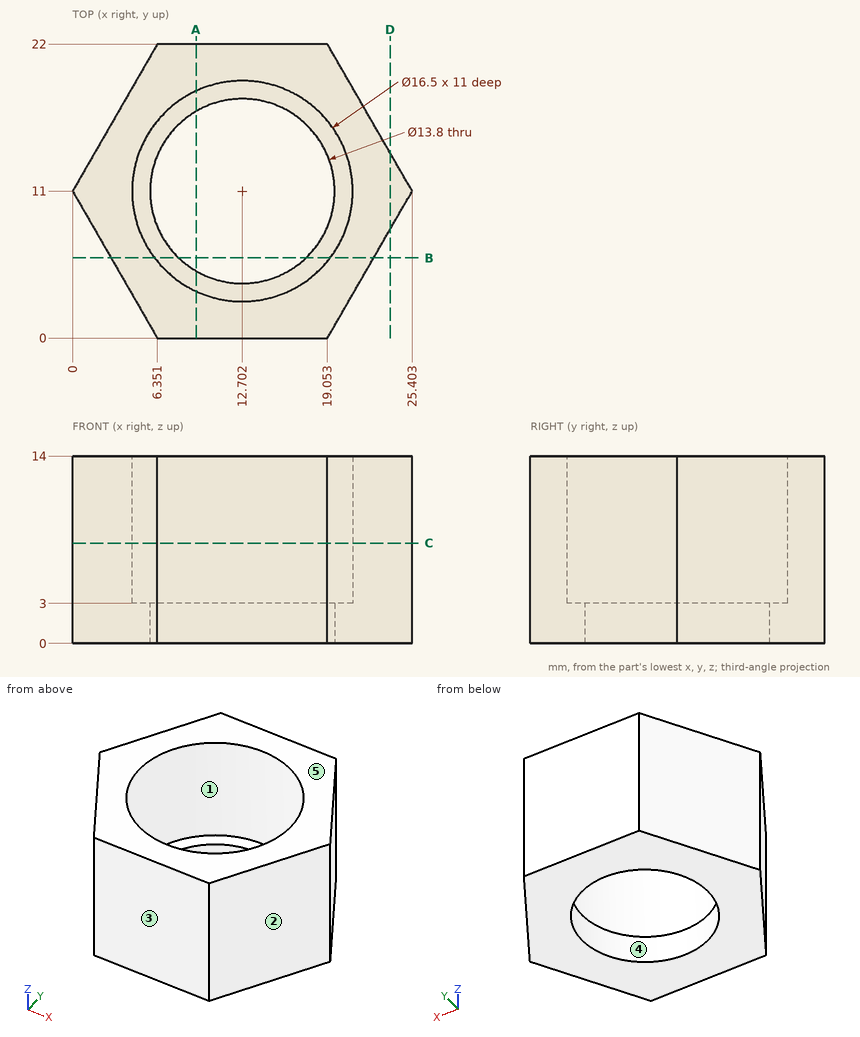
The drawing under review shows one solid part. Ordinate dimensions are in mm from its lowest x, y, z. A direction names the side the tool comes from. Coordinates: 2 decimals unless noted, no trailing zeros. Order: outer loops, then holes, each group sorted by start corner. A loop starts at its lowest first (then second) coordinate and runs counter-clockwise, first axis right, second up. Notation, with made-up numbers: (-35, -16) - (-29, -16) arc R24 ccw to (-29, 7) - close; hole circle Ø1 at (29.5, -30). An arc over 180 degrees is marked (long way). Put each result on its own line as item: value.
1) Wall thickness on L1, parallel to Y at x = 12, z = 5; L2, parallel to Z at x = 13, y = 4; L3, parallel to X at y = 13.25, z = 1.25 (1 decimal): over which ranges is each line inside the solid? List them lowest first. Write a range as from..to.
Response values:
L1: y = 0..2.78, 19.22..22
L2: z = 0..3
L3: x = 1.3..6.2, 19.2..24.1
2) Take a section at D-D, the plane x = 23.75. Give the boundary of the cut face in (y, z), and give its area (3 significant figures).
Response values:
outline: (8.14, 0) - (13.86, 0) - (13.86, 14) - (8.14, 14) - close
area: 80.2 mm²
3) The part is to be moulded in two halves that separate along Y. For the marked faces 3, 4 and 5, say which applies: released by +Y, released by -Y, zero draft, split by the parting line, or undercut.
Response values:
face 3: released by -Y
face 4: undercut
face 5: zero draft
4) Take a section at B-B, the plane y = 6. Give the boundary of the cut face in (x, z), and give its area (3 significant figures).
Response values:
outline: (2.89, 0) - (7.95, 0) - (7.95, 3) - (6.14, 3) - (6.14, 14) - (2.89, 14) - close; (17.46, 0) - (22.52, 0) - (22.52, 14) - (19.26, 14) - (19.26, 3) - (17.46, 3) - close
area: 102 mm²
5) Tool access review of the marked faces 1 and 2: name each direction out of +Z, -Z, +X, -X, +Y, -Y from which nothing blocks a thin tool from reaching the whole face with its end or side.
Response values:
face 1: +Z
face 2: +Z, -Z, +X, -Y
6) Take a section at C-C, the plane z = 7.5. Give the boundary of the cut face in (x, y), and give its area (3 significant figures).
Response values:
outline: (0, 11) - (6.35, 0) - (19.05, 0) - (25.4, 11) - (19.05, 22) - (6.35, 22) - close; hole circle Ø16.5 at (12.7, 11)
area: 205 mm²
7) Insertion check: P1, Ø3, axis at y = 4.5, z = 12, coming from the +X side; P2, Ø3, axis at y = 7.5, z = 12, coming from the +X side; P3, Ø13, axis at x = 12.7, y = 11, coming from the +Z side. Each pin has a flat end and moves straight along its axis. Give the tip position at first contact, or say it passes through.
Response values:
P1: stops at x = 22.52
P2: stops at x = 24.25
P3: passes through
8) Take a section at A-A, the plane x = 9.25. Give the boundary of the cut face in (y, z) (1 decimal), and give its area (3 significant figures).
Response values:
outline: (0, 0) - (5, 0) - (5, 3) - (3.5, 3) - (3.5, 14) - (0, 14) - close; (17, 0) - (22, 0) - (22, 14) - (18.5, 14) - (18.5, 3) - (17, 3) - close
area: 107 mm²
